The model under review builds one solid part; all positions refer to its coordinate system, in mm. A direction names the side the tool comes from. Round coordinates to 2 decimals unless told otherwise and drop trailing zeros. Order: outer loops, then holes, each group sorted by start corner. A loop starts at its lowest first (then second) coordinate and runs counter-clockwise, first axis right, second up. Notation, with made-up numbers: M 55,-6.75 L 99,-6.75 A13 cw 99,9.25 Z; hole C 49,-38.5 d6. An arc over 180 degrees is marked long. Answer as a JSON object with one key per item and string values. Group by question number.
1) Insertion check: pin 1 Ø2.5 at (x, y) = (1, 43) entering from +Z; pin 2 Ø2.5 at (x, y) = (13.2, 87.16) entering from +Z; pin 3 Ø2.5 at (x, y) = (0.1, 29.4) entering from +Z; pin 4 Ø0.6 at (x, z) = (2.5, 0) entering from +Y. Each pin has a flat end and moves straight along its axis. Give the tip position at first contact, or say it passes through.
2) The part is to be moulded in two halves that separate along Y. For faces 6 (the flat face through (16.2, 55.2, 0.3)), 7 (the flat face through (13.735, 78.244, -16.224)), 8 (the cylindrical face through (14.44, -7.49, 2.46)), say which applies: +Y half, -Y half, draft (parallel to the pull), parting line (faces both ways), or undercut.
3) To check wall thickness, follow line 1 (Z direction, x = 0, y = 89); line 2 (Y direction, x = 13.2, z = 3); line 3 (X direction, y = 81, z = -11.5). State the ranges of each line that lie inside material, in increasing order.
4) For faces 1 (the flat face through (0, 65, 2)), 2 (the cylindrical face through (-12.66, -8.13, 2.46)), 3 (the flat face through (0, 88, -32)), 4 (the flat face through (0, 89, 0.5)), 5 (the flat face through (0, 88, -8.3)), list the 3-axis set-ups (+Z, -Z, +X, -X, +Y, -Y) from which the entire face can be reached by the end or side of a thin tool; tool diameter is ignored.
5) Consider section A-A, the plane x = 10. Write out the cut boundary in (y, z), then the cut area to 3 significant figures.
6) Consider section D-D, the plane y = 7. Write out the cut boundary in (x, z), then the cut area to 3 significant figures.
Autodesk Inventor part; units mm, degrees
ref_plane "YZ Plane" through (0, 0, 0) normal (1, 0, 0) x (0, 1, 0)
ref_plane "XZ Plane" through (0, 0, 0) normal (0, 1, 0) x (-1, 0, 0)
ref_plane "XY Plane" through (0, 0, 0) normal (0, 0, 1) x (1, 0, 0)
ref_plane "Arbeitsebene1" through (0, 0, 0) normal (0, 0, 1) x (1, 0, 0)
sketch "Skizze1" plane through (0, 0, 0) normal (0, 0, 1) x (1, 0, 0)
  circle A0 centre (0.1, 41.9017) radius 1.75
  circle A1 centre (0.1, 29.4017) radius 1.75
  circle A2 centre (0.1, 16.9017) radius 1.75
  circle A3 centre (0.1, 4.4017) radius 1.75
  line L0 (6.05, 0) -> (-6.05, 0)
  line L1 (6.05, 0) -> (6.05, 50)
  line L2 (6.05, 50) -> (-6.05, 50)
  line L3 (-6.05, 0) -> (-6.05, 50)
  line L4 (13.5, 40.6086) -> (13.5, 8.2086)
  line L5 (-13.5, 40.6086) -> (-13.5, 8.2086)
  line L6 (13.5, -9.8404) -> (-13.3608, -9.8404)
  line L7 (-13.3608, -9.8404) -> (-13.3608, 90.1596)
  line L8 (-13.3608, 90.1596) -> (13.5, 90.1596)
  line L9 (13.5, 90.1596) -> (13.5, -9.8404)
  line L10 (-13.3608, 90.1596) -> (-16.2, 90.1596)
  line L11 (-16.2, 90.1596) -> (-16.2, -9.8404)
  line L12 (-16.2, -9.8404) -> (-13.3608, -9.8404)
  line L13 (-13.3608, -9.8404) -> (-13.3608, 90.1596)
  line L14 (13.5, -9.8404) -> (16.2, -9.8404)
  line L15 (16.2, -9.8404) -> (16.2, 90.1596)
  line L16 (16.2, 90.1596) -> (13.5, 90.1596)
  line L17 (13.5, 90.1596) -> (13.5, -9.8404)
  point P0 (0, 0)
  dimension "d0" = 100
  dimension "d34" = 27
  dimension "d35" = 2.7
  dimension "d36" = 2.7
extrude "Extrusion1" add sketch "Skizze1" along normal blind 5 contours A0 | A1 | A2 | A3 | L0 L3 L2 L1 | L9 L16 L15 L14 L4 | L4 L9 L6 L7 L8 | L7 L12 L11 L10
sketch "Skizze2" plane through (0, 0, 0) normal (0, 0, -1) x (-1, 0, 0)
  line L0 (-13.5, 90.1596) -> (16.2, 90.1596)
  line L1 (16.2, 90.1596) -> (-16.2, 90.1596)
  line L2 (-16.2, 90.1596) -> (-16.1921, 85.1596)
  line L3 (-16.1921, 85.1596) -> (16.2, 85.1596)
  line L4 (16.2, 85.1596) -> (16.2, 90.1596)
  line L5 (13.3608, -9.8404) -> (-13.5, -9.8404)
  line L6 (-13.5, -9.8404) -> (-13.5, -4.8404)
  line L7 (-13.5, -4.8404) -> (13.3608, -4.8404)
  line L8 (13.3608, -4.8404) -> (13.3608, -9.8404)
  line L9 (-16.2, 90.1596) -> (16.2, 90.1596)
  point P0 (0, 0)
  dimension "d3" = 5
  dimension "d4" = 5
extrude "Extrusion2" add sketch "Skizze2" along normal blind 32 contours L0 L4 L3 L2 L1
sketch "Skizze3" plane through (16.2, -9.8404, 5) normal (1, 0, 0) x (0, 0, -1)
  line L0 (5, 0) -> (5, 95)
  line L1 (5, 95) -> (37, 95)
  line L2 (37, 100) -> (37, 95)
  line L3 (37, 100) -> (0, 100)
  line L4 (0, 0) -> (0, 100)
  line L5 (37, 100) -> (37, 95)
  line L6 (37, 95) -> (5, 80.9723)
  line L7 (5, 95) -> (5, 5)
  line L8 (5, 0) -> (0, 0)
  point P0 (5, 9.8404)
extrude "Extrusion3" add sketch "Skizze3" against normal blind 5 contours L0 L1 L6
sketch "Skizze4" plane through (-16.2, -9.8404, 5) normal (-1, 0, 0) x (0, 0, 1)
  line L0 (-5, 95) -> (-5, 80.9723)
  line L1 (-37, 95) -> (-5, 95)
  line L2 (-37, 95) -> (-5, 80.9723)
  point P0 (-5, 9.8404)
extrude "Extrusion4" add sketch "Skizze4" against normal blind 5
sketch "Skizze5" plane through (11.2, 85.1596, -32) normal (0, -1, 0) x (1, 0, 0)
  circle A0 centre (-11.2, 4.1) radius 1.75
  point P0 (-11.2, 32)
hole "Bohrung1" at (0, 85.1596, -27.9) direction (0, 1, 0) diameter 3.2 end through all counterbore diameter 6 counterbore depth 3
sketch "Skizze6" plane through (0, 0, 5) normal (0, 0, 1) x (1, 0, 0)
  circle A0 centre (0.1, 16.9017) radius 1.75
  point P0 (0, 0)
hole "Bohrung2" at (0.1, 16.9017, 5) direction (0, 0, -1) diameter 3.2 end through all counterbore diameter 8 counterbore depth 3
pattern_linear "Rechteckige Anordnung1" count 6 spacing 12.5 along (0, 1, 0) count 2 spacing 12.5 along (0, -1, 0) of "Bohrung2"
sketch "Skizze7" plane through (-13.3608, 90.1596, 5) normal (0, 1, 0) x (1, 0, 0)
  arc A0 (19.4108, 9.1706) -> (19.209, 9.3127) centre (19.1621, 9.0317) ccw
  arc A1 (18.9122, 9.7059) -> (19.209, 9.3127) centre (19.9951, 10.2147) ccw
  arc A2 (18.9122, 9.7059) -> (18.7859, 9.8171) centre (18.694, 9.5854) ccw
  line L0 (18.7859, 9.8171) -> (18.2888, 9.8559)
  arc A3 (18.0608, 10.0745) -> (18.2888, 9.8559) centre (18.3083, 10.1044) ccw
  line L1 (18.0608, 10.0745) -> (18.0608, 10.5256)
  arc A4 (18.2884, 10.7739) -> (18.0608, 10.5256) centre (18.3101, 10.5256) ccw
  line L2 (18.2884, 10.7739) -> (18.6539, 10.8058)
  arc A5 (18.6539, 10.8058) -> (18.9122, 10.9588) centre (18.6817, 11.0536) ccw
  arc A6 (19.2562, 11.4767) -> (18.9122, 10.9588) centre (20.0633, 10.5674) ccw
  arc A7 (19.2562, 11.4767) -> (19.4108, 11.7) centre (19.1617, 11.7073) ccw
  line L3 (19.4108, 11.7) -> (19.4108, 12.3)
  line L4 (19.4108, 12.3) -> (18.9108, 12.8)
  line L5 (18.9108, 12.8) -> (7.8108, 12.8)
  line L6 (7.3108, 12.3) -> (7.8108, 12.8)
  line L7 (7.3108, 11.7) -> (7.3108, 12.3)
  arc A8 (7.3108, 11.7) -> (7.4655, 11.4767) centre (7.56, 11.7073) ccw
  arc A9 (7.8095, 10.9588) -> (7.4655, 11.4767) centre (6.6584, 10.5674) ccw
  arc A10 (7.8095, 10.9588) -> (8.0678, 10.8058) centre (8.04, 11.0536) ccw
  line L8 (8.4333, 10.7739) -> (8.0678, 10.8058)
  arc A11 (8.6608, 10.5256) -> (8.4333, 10.7739) centre (8.4116, 10.5256) ccw
  line L9 (8.6608, 10.0745) -> (8.6608, 10.5256)
  arc A12 (8.4328, 9.8559) -> (8.6608, 10.0745) centre (8.4134, 10.1044) ccw
  line L10 (7.9358, 9.8171) -> (8.4328, 9.8559)
  arc A13 (7.9358, 9.8171) -> (7.8095, 9.7059) centre (8.0277, 9.5854) ccw
  arc A14 (7.5127, 9.3127) -> (7.8095, 9.7059) centre (6.7266, 10.2147) ccw
  arc A15 (7.5127, 9.3127) -> (7.3108, 9.1706) centre (7.5596, 9.0317) ccw
  line L11 (7.3108, 5) -> (7.3108, 9.1706)
  line L12 (19.4108, 5) -> (7.3108, 5)
  line L13 (19.4108, 5) -> (19.4108, 9.1706)
  arc A16 (19.9108, 9.2672) -> (19.475, 9.7515) centre (19.1621, 9.0317) ccw
  arc A17 (19.3606, 9.9276) -> (19.475, 9.7515) centre (19.9951, 10.2147) ccw
  arc A18 (19.3606, 9.9276) -> (18.8795, 10.3114) centre (18.694, 9.5854) ccw
  line L14 (18.8795, 10.3114) -> (18.8155, 10.3163)
  arc A19 (18.8155, 10.3163) -> (19.3826, 10.7888) centre (18.6817, 11.0536) ccw
  arc A20 (19.5506, 11.0669) -> (19.3826, 10.7888) centre (20.0633, 10.5674) ccw
  arc A21 (19.5506, 11.0669) -> (19.9108, 11.6946) centre (19.1617, 11.7073) ccw
  line L15 (19.9108, 11.6946) -> (19.9108, 12.5071)
  line L16 (19.9108, 12.5071) -> (19.118, 13.3)
  line L17 (19.118, 13.3) -> (7.6037, 13.3)
  line L18 (7.6037, 13.3) -> (6.8108, 12.5071)
  line L19 (6.8108, 12.5071) -> (6.8108, 11.6946)
  arc A22 (6.8108, 11.6946) -> (7.1711, 11.0669) centre (7.56, 11.7073) ccw
  arc A23 (7.3391, 10.7888) -> (7.1711, 11.0669) centre (6.6584, 10.5674) ccw
  arc A24 (7.3391, 10.7888) -> (7.9062, 10.3163) centre (8.04, 11.0536) ccw
  line L20 (7.9062, 10.3163) -> (7.8422, 10.3114)
  arc A25 (7.8422, 10.3114) -> (7.3611, 9.9276) centre (8.0277, 9.5854) ccw
  arc A26 (7.2467, 9.7515) -> (7.3611, 9.9276) centre (6.7266, 10.2147) ccw
  arc A27 (7.2467, 9.7515) -> (6.8108, 9.2672) centre (7.5596, 9.0317) ccw
  line L21 (6.8108, 9.2672) -> (6.8108, 4.5)
  line L22 (6.8108, 4.5) -> (19.9108, 4.5)
  line L23 (19.9108, 4.5) -> (19.9108, 9.2672)
  point P0 (13.3608, 5)
  dimension "d31" = 0.5
extrude "Extrusion5" cut sketch "Skizze7" against normal up to surface (5 mm away) contours L13 L12 L11 A15 A14 A13 L10 A12 L9 A11 L8 A10 A9 A8 L7 L6 L5 L4 L3 A7 A6 A5 L2 A4 L1 A3 L0 A2 A1 A0 | L23 L22 L21 A27 A26 A25 L20 A24 A23 A22 L19 L18 L17 L16 L15 A21 A20 A19 L14 A18 A17 A16
sketch "Skizze10" plane through (0, 0, 5) normal (0, 0, 1) x (1, 0, 0)
  line L0 (16.2, -9.8404) -> (16.2, 90.1596)
  line L1 (-16.2, 90.1596) -> (-16.2, -9.8404)
  line L2 (16.2, 90.1596) -> (-16.2, 90.1596)
  line L3 (-13.2, 54.7596) -> (13.2, 54.7596)
  line L4 (13.2, 54.7596) -> (13.2, 87.1596)
  line L5 (13.2, 87.1596) -> (-13.2, 87.1596)
  line L6 (-13.2, 87.1596) -> (-13.2, 54.7596)
  line L7 (-13.2, 54.7596) -> (13.2, 87.1596) construction
  line L8 (13.2, 54.7596) -> (-13.2, 87.1596) construction
  line L9 (18.5, 39.0086) -> (18.5, 36.2086)
  line L10 (17.2, 28.5596) -> (-15.2, 28.5596)
  line L11 (-13.2, -6.8404) -> (13.2, -6.8404)
  line L12 (13.2, -6.8404) -> (13.2, 25.5596)
  line L13 (13.2, 25.5596) -> (-13.2, 25.5596)
  line L14 (-13.2, 25.5596) -> (-13.2, -6.8404)
  line L15 (-13.2, -6.8404) -> (13.2, 25.5596) construction
  line L16 (13.2, -6.8404) -> (-13.2, 25.5596) construction
  line L17 (18.5, 40.6086) -> (18.5, 8.2086)
  point P0 (0, 0)
  point P1 (0, 70.9596)
  point P2 (0, 87.1596)
  point P3 (0, 9.3596)
  point P4 (0, 25.5596)
  dimension "d37" = 26.4
  dimension "d38" = 32.4
  dimension "d39" = 3
  dimension "d47" = 26.4
  dimension "d48" = 32.4
  dimension "d49" = 3
  dimension "d50" = 3
hole "Bohrung3" at (0, 87.1596, 5) at (13.2, 54.7596, 5) at (-13.2, 54.7596, 5) at (-13.2, 87.1596, 5) at (13.2, 87.1596, 5) at (-13.2, -6.8404, 5) at (13.2, -6.8404, 5) at (13.2, 25.5596, 5) at (-13.2, 25.5596, 5) direction (0, 0, -1) diameter 2.8 depth 8 tip angle 118
equation "\"d36\" = d35"
properties part number "30_Linear_Captive_Nema8_Base"
Results list:
{
 "1": {"pin 1": "z = 2", "pin 2": "z = -3.09", "pin 3": "through", "pin 4": "y = 85.16"},
 "2": {"face 6": "draft", "face 7": "-Y half", "face 8": "undercut"},
 "3": {"line 1": "-32 to -29.5, -26.3 to -8.3, 0.5 to 5", "line 2": "-9.84 to -8.24, -5.44 to 24.16, 26.96 to 53.36, 56.16 to 85.76, 88.56 to 90.16", "line 3": "-16.2 to -11.2, 11.2 to 16.2"},
 "4": {"face 1": "+Z", "face 2": "+Z, -Z", "face 3": "-Z, +X, -X, +Y, -Y", "face 4": "+Y", "face 5": "+Y, -Y"},
 "5": {"outline": "M -9.84,0 L 85.16,0 L 85.16,-32 L 90.16,-32 L 90.16,5 L -9.84,5 Z", "area": "660 mm^2"},
 "6": {"outline": "M -16.2,0 L 16.2,0 L 16.2,5 L 3.14,5 L 3.14,2 L -2.94,2 L -2.94,5 L -16.2,5 Z", "area": "144 mm^2"}
}
